Here's how the part is built. I have some questions about the finished solid (model axes, mm). Face numbers are marked on the shaded views. Coordinates: 2 decimals unless noted, no trailing zeros. Write each loop counter-clockwise with the first axis right and the second up, starting at its lowest first coordinate (ties: lowest second). Pieces come first, ordered by that corner, then holes.
Item 1: I'm going to push flat-ended pins straight in: P1, Ø10, axis at x = 93, z = 5.5, coming from the -Y side; P2, Ø1.5, axis at x = 94.5, z = 2, coming from the -Y side; P3, Ø3, axis at x = 77.5, z = -5.5, coming from the -Y side. Where does each tip first touch, or does it pass through?
Item 2: If we mould it in two halves opening along Y, with no side actions, what happens to the marked faces 1, 2 and 3? For each: pulls with the +Y half, pulls with the -Y half, needs draft (parallel to the pull), parting line crosses it, or undercut.
Item 3: I want a section at A-A (x = 85). Please give me the cut outline in (y, z), and give its area (3 significant figures).
Item 4: I want a section at C-C (z = -18). Please give me the cut outline in (x, y), and give its area (3 significant figures).
Item 5: I want a section at B-B (y = 14.5). Please give me the cut outline in (x, z).
Item 6: Please list where these lines run through material, in increasing order: line 1 (Z direction, x = 46, y = 6.5); line 2 (Y direction, x = 112.5, z = 2.5); line 3 (Y direction, x = 50, z = 10.5).
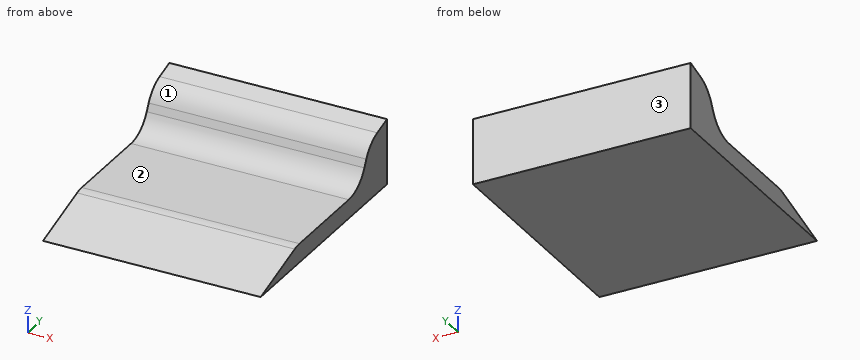
from build123d import *

# Parameters (mm, degrees)
F1_DEPTH = 133
F2_R     = 20


with BuildPart() as f1:
    # F0 (on Right) → F1 (new body)
    with BuildSketch(Plane.YZ):
        Polygon((-31.488675, -9.528097), (-72.819769, -21.046512), (70.710715, -21.046512), (70.710715, 18.953488), (51.226363, 13.523463), (39.479751, -9.528097), align=None)
    extrude(amount=F1_DEPTH)

    # F2
    f2_edges = [f1.edges().sort_by_distance(p)[0] for p in [
        (66.5, 39.479751, -9.528097),
        (66.5, -31.488675, -9.528097),
        (66.5, 51.226363, 13.523463),
    ]]
    fillet(f2_edges, radius=F2_R)


solid = f1.part
Answer:
1. P1: stops at y = 44.56
1. P2: stops at y = 44.97
1. P3: stops at y = 36.96
2. face 1: pulls with the -Y half
2. face 2: needs draft
2. face 3: pulls with the +Y half
3. outline: (-72.82, -21.05) - (70.71, -21.05) - (70.71, 18.95) - (59.69, 15.88) arc R20 ccw to (47.24, 5.7) - (45.04, 1.39) arc R20 cw to (27.22, -9.53) - (-28.75, -9.53) arc R20 ccw to (-34.12, -10.26) - close
3. area: 2,070 mm2
4. outline: (0, -61.89) - (133, -61.89) - (133, 70.71) - (0, 70.71) - close
4. area: 17,600 mm2
5. outline: (0, -21.05) - (133, -21.05) - (133, -9.53) - (0, -9.53) - close
6. line 1: z = -21.05 to -9.53
6. line 2: y = 45.61 to 70.71
6. line 3: y = 50.66 to 70.71
